Check sheet for the modelled part. Datum: model origin and axes. Units: mm. A direction names the side the tool comes from. Give positions to 0.01 mm unless a question says otherwise; leave off trailing zeros. Loops run counter-clockwise (first coordinate to the right, second up) from the corner with the lowest first, then second, coordinate; pieces in that order, holes last.
```python
from build123d import *

# Parameters (mm, degrees)
F1_DEPTH = 38.1
F2_R     = 5.020129
F3_DEPTH = 24.13


with BuildPart() as f1:
    # F0 (on Right) → F1 (new body)
    with BuildSketch(Plane.YZ):
        Polygon((21.585431, 43.170862), (0, 43.170862), (0, 0), (43.170862, 0), (43.170862, 14.348196), (21.585431, 14.348196), align=None)
    extrude(amount=F1_DEPTH)

    # F2 (on face) → F3 (cut)
    with BuildSketch(Plane(origin=(0, 21.585431, 0), x_dir=(-1, 0, 0), z_dir=(0, 1, 0))):
        with Locations((-19.150337, 36.581956)):
            Circle(F2_R)
    extrude(amount=-F3_DEPTH, mode=Mode.SUBTRACT)


solid = f1.part
```
(1) Gauge pin test, flat ends, axial feed: pin 1 Ø6 at (x, z) = (19.15, 36.58) entering from +Y; pin 2 Ø14.5 at (x, z) = (17.5, 27) entering from +Y; pin 3 Ø6.5 at (x, y) = (10.5, 29.5) entering from +Z. Record the tip position at first contact, or that the pin passes through.
(2) Section check D-D on x = 30.5. Record the boundary of the cut face in (y, z).
(3) Release check for a two-part mould opening along Z. For faces 1 (the face through (16.452, 10.944, 40.815)), 2 (the face through (19, 33, 14.348)), 3 (the face through (0, 16, 17)) record: pulls with the +Z half, pulls with the -Z half, needs draft (parallel to the pull), parting line crosses it, or undercut.
(4) Section check B-B on x = 18.5. Record the boundary of the cut face in (y, z), plus the area to 3 significant figures.
(5) Material ranges on line 1 (Y direction, x = 4.5, z = 19); line 2 (Z direction, x = 29.5, y = 35); line 3 (X direction, y = 4, z = 35), recorded low to high.
(6) Access from +Z, -Z, +X, -X, +Y, -Y to the whole of each face (thin tool, end or side, straight path). Record for faces 4 (the face through (19, 43.171, 7)), 5 (the face through (19, 21.585, 29)).
(7) Section check A-A on z = 35. Record the boundary of the cut face in (x, y), plus the area to 3 significant figures.
(8) Section check C-C on y = 21. Record the boundary of the cut face in (x, z).
Computed values:
1. pin 1: passes through
1. pin 2: stops at y = 21.59
1. pin 3: stops at z = 14.35
2. outline: (0, 0) - (43.17, 0) - (43.17, 14.35) - (21.59, 14.35) - (21.59, 43.17) - (0, 43.17) - close
3. face 1: undercut
3. face 2: pulls with the +Z half
3. face 3: needs draft
4. outline: (0, 0) - (43.17, 0) - (43.17, 14.35) - (21.59, 14.35) - (21.59, 31.6) - (0, 31.6) - close; (0, 41.56) - (21.59, 41.56) - (21.59, 43.17) - (0, 43.17) - close
4. area: 1,030 mm2
5. line 1: y = 0 to 21.59
5. line 2: z = 0 to 14.35
5. line 3: x = 0 to 14.39, 23.91 to 38.1
6. face 4: +Z, -Z, +X, -X, +Y
6. face 5: +Z, +X, -X, +Y
7. outline: (0, 0) - (14.39, 0) - (14.39, 21.59) - (0, 21.59) - close; (23.91, 0) - (38.1, 0) - (38.1, 21.59) - (23.91, 21.59) - close
7. area: 617 mm2
8. outline: (0, 0) - (38.1, 0) - (38.1, 43.17) - (0, 43.17) - close; hole circle Ø10.04 at (19.15, 36.58)
